```python
from build123d import *

# Parameters (mm, degrees)
SKETCH1_R                = 1.5
SKETCH1_R_2              = 2.5
BOSS_EXTRUDE1_DEPTH      = 20
SKETCH2_W                = 8.1
SKETCH2_H                = 20
SKETCH2_W_2              = 5.2
SKETCH2_W_3              = 5.1
CUT_EXTRUDE1_DEPTH       = 20
CUT_EXTRUDE1_DEPTH_BACK  = 20
CUT_EXTRUDE2_DEPTH       = 9
BOSS_EXTRUDE2_DEPTH      = 11.9
SKETCH5_R                = 3
BOSS_EXTRUDE3_DEPTH      = 5
CUT_EXTRUDE6_DEPTH       = 1
SKETCH13_R               = 2.5
CUT_EXTRUDE7_DEPTH       = 4
BOSS_EXTRUDE4_DEPTH      = 3
CUT_EXTRUDE9_DEPTH       = 3
SKETCH17_W               = 9
SKETCH17_H               = 3.569322199
CUT_EXTRUDE11_DEPTH      = 3
SKETCH18_W               = 5.770974844
SKETCH18_H               = 0.772936936
BOSS_EXTRUDE5_DEPTH      = 6.9
BOSS_EXTRUDE5_DEPTH_BACK = 1
SKETCH19_W               = 5.1
SKETCH19_H               = 16.397725614
CUT_EXTRUDE12_DEPTH      = 0.301495
SKETCH20_W               = 5
SKETCH20_H               = 12.419235667
CUT_EXTRUDE13_DEPTH      = 10
BOSS_EXTRUDE6_DEPTH      = 2
SKETCH23_W               = 4.9
SKETCH23_H               = 6
BOSS_EXTRUDE7_DEPTH      = 4
SKETCH22_R               = 1
CUT_EXTRUDE15_DEPTH      = 8
BOSS_EXTRUDE8_DEPTH      = 2
SKETCH14_R               = 1.5
CUT_EXTRUDE8_DEPTH       = 10.1
CUT_EXTRUDE17_DEPTH      = 8.1
CUT_EXTRUDE17_DEPTH_BACK = 2
CUT_EXTRUDE18_DEPTH      = 2
CUT_EXTRUDE20_DEPTH      = 5.2
SKETCH30_W               = 6.9
SKETCH30_H               = 20
CUT_EXTRUDE21_DEPTH      = 0.283797
CUT_EXTRUDE22_REACH      = 91.699
SKETCH31_W               = 2
SKETCH31_H               = 11.022421386
CUT_EXTRUDE23_DEPTH      = 7
CUT_EXTRUDE24_DEPTH      = 21
SKETCH34_W               = 60.526432738
SKETCH34_H               = 58.455185991
CUT_EXTRUDE25_DEPTH      = 21


with BuildPart() as part:
    # Sketch1 → Boss-Extrude1 (new body)
    with BuildSketch(Plane(origin=(0, 0, 0), x_dir=(0, 0, -1), z_dir=(1, 0, 0))):
        with BuildLine():
            ThreePointArc((9.765353557, 20.116545894), (0, 32.270117322), (-9.765353557, 20.116545894))
            ThreePointArc((-9.765353557, 20.116545894), (-5.132645827, -18.047253777), (-7.88740095, -56.392382678))
            ThreePointArc((-7.88740095, -56.392382678), (0, -65.729882678), (7.88740095, -56.392382678))
            ThreePointArc((7.88740095, -56.392382678), (5.132645827, -18.047253777), (9.765353557, 20.116545894))
        make_face()
        with Locations((0, 22.270117322)):
            Circle(SKETCH1_R, mode=Mode.SUBTRACT)
        with Locations((0, -57.729882678)):
            Circle(SKETCH1_R_2, mode=Mode.SUBTRACT)
    extrude(amount=BOSS_EXTRUDE1_DEPTH)

    # Sketch2 → Cut-Extrude1 (cut, two sides)
    with BuildSketch(Plane.XY) as cut_extrude1_sk:
        with Locations((4.05, -55.729882678)):
            Rectangle(SKETCH2_W, SKETCH2_H)
        with Locations((17.4, -55.729882678)):
            Rectangle(SKETCH2_W_2, SKETCH2_H)
        with Locations((5.55, 22.270117322)):
            Rectangle(SKETCH2_W_3, SKETCH2_H)
    extrude(amount=CUT_EXTRUDE1_DEPTH, mode=Mode.SUBTRACT)
    extrude(cut_extrude1_sk.sketch, amount=-CUT_EXTRUDE1_DEPTH_BACK, mode=Mode.SUBTRACT)

    # Sketch3 → Cut-Extrude2 (cut)
    with BuildSketch(Plane.ZY.offset(-8.1)):
        with BuildLine():
            Line((8.5, 22.270117322), (8.5, 40.909533312))
            Line((8.5, 40.909533312), (-17.52872033, 40.909533312))
            Line((-17.52872033, 40.909533312), (-17.52872033, 13.770117322))
            Line((-17.52872033, 13.770117322), (0, 13.770117322))
            ThreePointArc((0, 13.770117322), (6.01040764, 16.259709682), (8.5, 22.270117322))
        make_face()
    extrude(amount=-CUT_EXTRUDE2_DEPTH, mode=Mode.SUBTRACT)

    # Sketch4 → Boss-Extrude2 (add, through all)
    with BuildSketch(Plane.ZY.offset(-8.1)):
        Polygon((8.5, 27.537944199), (8.283796844, 12.741558936), (10.283796844, 12.741558936), (10.283796844, 27.537944199), align=None)
    extrude(amount=-BOSS_EXTRUDE2_DEPTH)

    # Sketch5 → Boss-Extrude3 (add)
    with BuildSketch(Plane.ZY.offset(-8.1)):
        with BuildLine():
            Line((8.145156861, 11.968622), (8.447845456, 23.968622))
            Line((8.447845456, 23.968622), (9.854698466, 23.968622))
            Line((9.854698466, 23.968622), (15.022421386, 23.968622))
            ThreePointArc((15.022421386, 23.968622), (21.022421386, 17.968622), (15.022421386, 11.968622))
            Line((15.022421386, 11.968622), (8.145156861, 11.968622))
        make_face()
        with Locations((15.022421386, 17.968622)):
            Circle(SKETCH5_R, mode=Mode.SUBTRACT)
    extrude(amount=-BOSS_EXTRUDE3_DEPTH)

    # Sketch12 → Cut-Extrude6 (cut)
    with BuildSketch(Plane(origin=(13.1, 0, 0), x_dir=(0, 0, -1), z_dir=(1, 0, 0))):
        Polygon((-13.902900694, 14.968622), (-13.902900694, 12.968622), (-15.902900694, 12.968622), (-15.902900694, 14.968622), (-15.902900694, 15.294296094), (-13.902900694, 15.294296094), align=None)
    extrude(amount=-CUT_EXTRUDE6_DEPTH, mode=Mode.SUBTRACT)

    # Sketch13 → Cut-Extrude7 (cut)
    with BuildSketch(Plane.ZY.offset(-17.1)):
        with Locations((0, 22.270117322)):
            Circle(SKETCH13_R)
    extrude(amount=-CUT_EXTRUDE7_DEPTH, mode=Mode.SUBTRACT)

    # Sketch15 → Boss-Extrude4 (add)
    with BuildSketch(Plane.ZY):
        Polygon((10, 22.270117322), (10, 11.968622), (8.145156861, 11.968622), (7.595672539, 11.968622), align=None)
    extrude(amount=-BOSS_EXTRUDE4_DEPTH)

    # Sketch16 → Cut-Extrude9 (cut)
    with BuildSketch(Plane(origin=(20, 0, 0), x_dir=(0, 0, -1), z_dir=(1, 0, 0))):
        with BuildLine():
            Line((-10.283796844, 23.968622), (-9.854698466, 23.968622))
            ThreePointArc((-9.854698466, 23.968622), (-9.349264901, 25.818531871), (-8.5, 27.537944199))
            Line((-8.5, 27.537944199), (-10.283796844, 27.537944199))
            Line((-10.283796844, 27.537944199), (-10.283796844, 23.968622))
        make_face()
    extrude(amount=-CUT_EXTRUDE9_DEPTH, mode=Mode.SUBTRACT)

    # Sketch17 → Cut-Extrude11 (cut)
    with BuildSketch(Plane.XY.offset(10.283796844)):
        with Locations((12.6, 25.7532831)):
            Rectangle(SKETCH17_W, SKETCH17_H)
    extrude(amount=-CUT_EXTRUDE11_DEPTH, mode=Mode.SUBTRACT)

    # Sketch18 → Boss-Extrude5 (add, two sides)
    with BuildSketch(Plane(origin=(13.1, 0, 0), x_dir=(0, 0, -1), z_dir=(1, 0, 0))) as boss_extrude5_sk:
        with Locations((-7.398309422, 12.355090468)):
            Rectangle(SKETCH18_W, SKETCH18_H)
    extrude(amount=BOSS_EXTRUDE5_DEPTH)
    extrude(boss_extrude5_sk.sketch, amount=-BOSS_EXTRUDE5_DEPTH_BACK)

    # Sketch19 → Cut-Extrude12 (cut)
    with BuildSketch(Plane(origin=(0, 12.270117322, 0), x_dir=(1, 0, 0), z_dir=(0, 1, 0))):
        with Locations((5.55, 0)):
            Rectangle(SKETCH19_W, SKETCH19_H)
    extrude(amount=-CUT_EXTRUDE12_DEPTH, mode=Mode.SUBTRACT)

    # Sketch20 → Cut-Extrude13 (cut)
    with BuildSketch(Plane.ZY.offset(-17.1)):
        with Locations((0, 28.479735156)):
            Rectangle(SKETCH20_W, SKETCH20_H)
    extrude(amount=-CUT_EXTRUDE13_DEPTH, mode=Mode.SUBTRACT)

    # Sketch21 → Boss-Extrude6 (add)
    with BuildSketch(Plane.ZY.offset(-17.1)):
        with BuildLine():
            Line((-8.473151119, 13.770117322), (0.278481736, 12.273995678))
            ThreePointArc((0.278481736, 12.273995678), (9.936881703, 21.148341047), (2.5, 31.952575688))
            Line((2.5, 31.952575688), (2.5, 22.270117322))
            ThreePointArc((2.5, 22.270117322), (0, 19.770117322), (-2.5, 22.270117322))
            Line((-2.5, 22.270117322), (-2.5, 31.952575688))
            ThreePointArc((-2.5, 31.952575688), (-8.522477621, 27.501501002), (-9.765353557, 20.116545894))
            ThreePointArc((-9.765353557, 20.116545894), (-9.093560923, 16.948562662), (-8.473151119, 13.770117322))
        make_face()
    extrude(amount=BOSS_EXTRUDE6_DEPTH)

    # Sketch23 → Boss-Extrude7 (add)
    with BuildSketch(Plane.XY.offset(10.283796844)):
        with Locations((17.55, 26.968622)):
            Rectangle(SKETCH23_W, SKETCH23_H)
    extrude(amount=-BOSS_EXTRUDE7_DEPTH)

    # Sketch22 → Cut-Extrude15 (cut)
    with BuildSketch(Plane.XY.offset(10.283796844)):
        with Locations((17.55, 26.870117322)):
            Circle(SKETCH22_R)
    extrude(amount=-CUT_EXTRUDE15_DEPTH, mode=Mode.SUBTRACT)

    # Sketch24 → Boss-Extrude8 (add)
    with BuildSketch(Plane.ZY.offset(-8.1)):
        with BuildLine():
            Line((5.147845456, 19.737443909), (5.147845456, 15.506265819))
            Line((5.147845456, 15.506265819), (8.447845456, 15.506265819))
            Line((8.447845456, 15.506265819), (8.447845456, 23.968622))
            add(Edge.make_bspline(
                [(8.447845456, 23.968622), (5.147845456, 23.968622), (5.147845456, 19.737443909)],
                knots=[3.141592654, 3.141592654, 3.141592654, 4.71238898, 4.71238898, 4.71238898], degree=2, weights=[1, 0.707106781, 1]))
        make_face()
    extrude(amount=-BOSS_EXTRUDE8_DEPTH)

    # Sketch14 → Cut-Extrude8 (cut)
    with BuildSketch(Plane.ZY):
        with Locations((7.532575614, 18.331804915)):
            Circle(SKETCH14_R)
    extrude(amount=-CUT_EXTRUDE8_DEPTH, mode=Mode.SUBTRACT)

    # Sketch25 → Cut-Extrude17 (cut, two sides)
    with BuildSketch(Plane.ZY.offset(-8.1)) as cut_extrude17_sk:
        with BuildLine():
            Line((12, -45.729882678), (8.346153846, -36.960651908))
            ThreePointArc((8.346153846, -36.960651908), (6.973852263, -42.37911752), (2.5, -45.729882678))
            Line((2.5, -45.729882678), (2.5, -53.227383372))
            ThreePointArc((2.5, -53.227383372), (0, -62.879882678), (-2.5, -53.227383372))
            Line((-2.5, -53.227383372), (-2.5, -45.729882678))
            ThreePointArc((-2.5, -45.729882678), (-6.973852263, -42.37911752), (-8.346153846, -36.960651908))
            Line((-8.346153846, -36.960651908), (-12, -45.729882678))
            Line((-12, -45.729882678), (-12, -57.729882678))
            ThreePointArc((-12, -57.729882678), (0, -69.729882678), (12, -57.729882678))
            Line((12, -57.729882678), (12, -45.729882678))
        make_face()
    extrude(amount=CUT_EXTRUDE17_DEPTH, mode=Mode.SUBTRACT)
    extrude(cut_extrude17_sk.sketch, amount=-CUT_EXTRUDE17_DEPTH_BACK, mode=Mode.SUBTRACT)

    # Sketch26 → Cut-Extrude18 (cut)
    with BuildSketch(Plane(origin=(20, 0, 0), x_dir=(0, 0, -1), z_dir=(1, 0, 0))):
        with BuildLine():
            Line((-7.209968303, 15.085404497), (-10.283796844, 15.085404497))
            Line((-10.283796844, 15.085404497), (-10.283796844, 17.085404497))
            Line((-10.283796844, 17.085404497), (-7.209968303, 17.085404497))
            ThreePointArc((-7.209968303, 17.085404497), (-4.010444351, 15.949526558), (-2.243391617, 13.050441039))
            ThreePointArc((-2.243391617, 13.050441039), (0.649659998, -12.257973546), (0.397031114, -37.729953741))
            Line((0.397031114, -37.729953741), (-1.608183929, -37.729953741))
            ThreePointArc((-1.608183929, -37.729953741), (-1.343036313, -12.450773719), (-4.206611504, 12.667092093))
            ThreePointArc((-4.206611504, 12.667092093), (-5.281990934, 14.405678614), (-7.209968303, 15.085404497))
        make_face()
    extrude(amount=-CUT_EXTRUDE18_DEPTH, mode=Mode.SUBTRACT)

    # Sketch29 → Cut-Extrude20 (cut)
    with BuildSketch(Plane(origin=(20, 0, 0), x_dir=(0, 0, -1), z_dir=(1, 0, 0))):
        with BuildLine():
            Line((8, -37.729882678), (8.140336581, -37.729882678))
            Line((8.140336581, -37.729882678), (8.140336581, -45.937498976))
            Line((8.140336581, -45.937498976), (-15.754893946, -45.937498976))
            Line((-15.754893946, -45.937498976), (-15.754893946, -37.729882678))
            Line((-15.754893946, -37.729882678), (-8, -37.729882678))
            ThreePointArc((-8, -37.729882678), (0, -45.729882678), (8, -37.729882678))
        make_face()
    extrude(amount=-CUT_EXTRUDE20_DEPTH, mode=Mode.SUBTRACT)

    # Sketch30 → Cut-Extrude21 (cut)
    with BuildSketch(Plane.XY.offset(10.283796844)):
        with Locations((16.55, 21.968622)):
            Rectangle(SKETCH30_W, SKETCH30_H)
    extrude(amount=-CUT_EXTRUDE21_DEPTH, mode=Mode.SUBTRACT)

    # Sketch31 → Cut-Extrude22 (cut, up to next)
    with BuildSketch(Plane(origin=(0, 23.968622, 0), x_dir=(1, 0, 0), z_dir=(0, 1, 0)), mode=Mode.PRIVATE) as cut_extrude22_sk1:
        with Locations((9.1, -15.511210693)):
            Rectangle(SKETCH31_W, SKETCH31_H)
    cut_extrude22_tool1 = extrude(cut_extrude22_sk1.sketch, amount=-CUT_EXTRUDE22_REACH, mode=Mode.PRIVATE) & part.part
    add(cut_extrude22_tool1.solids().sort_by_distance((9.1, 23.968622, 15.511211))[0], mode=Mode.SUBTRACT)

    # Sketch32 → Cut-Extrude23 (cut)
    with BuildSketch(Plane.ZY.offset(-8.1)):
        Polygon((-8.473151119, 13.770117322), (-8.473151119, 5.401068454), (5.147845456, 15.506265819), align=None)
    extrude(amount=-CUT_EXTRUDE23_DEPTH, mode=Mode.SUBTRACT)

    # Sketch33 → Cut-Extrude24 (cut, through all)
    with BuildSketch(Plane(origin=(20, 0, 0), x_dir=(0, 0, -1), z_dir=(1, 0, 0))):
        Polygon((-9.30475326, -22.954882678), (-9.30475326, -27.954882678), (8.892389241, -27.954882678), (8.892389241, -22.954882678), (8.892389241, -17.954882678), (-9.30475326, -17.954882678), align=None)
    extrude(amount=-CUT_EXTRUDE24_DEPTH, mode=Mode.SUBTRACT)

    # Sketch34 → Cut-Extrude25 (cut, through all)
    with BuildSketch(Plane(origin=(20, 0, 0), x_dir=(0, 0, -1), z_dir=(1, 0, 0))):
        with Locations((-5.515206789, -53.322694673)):
            Rectangle(SKETCH34_W, SKETCH34_H)
    extrude(amount=-CUT_EXTRUDE25_DEPTH, mode=Mode.SUBTRACT)


solid = part.part
```
Verification items for the finished model (mm, model axes). A direction names the side the tool comes from. Round coordinates to 2 decimals unless told otherwise and drop trailing zeros. Order: outer loops, then holes, each group sorted by start corner. A loop starts at its lowest first (then second) coordinate and runs counter-clockwise, first axis right, second up.
1) Draft check along X on faces 5 (the flat face through (3, 20, 0)), 6 (the flat face through (0, 8, 0)), 7 (the flat face through (1, 11.969, 9)). Enter one of: +X half, -X half, draft (parallel to the pull), parting line (faces both ways), or undercut.
Geometry says:
face 5: undercut
face 6: -X half
face 7: draft
2) Material ranges on line 1 (Y direction, x = 0.8, z = 0); line 2 (X direction, y = 20, z = 4); line 3 (Y direction, x = 8, z = 1.5), recorded low to high.
Geometry says:
line 1: y = -17.95 to 20.77, 23.77 to 32.27
line 2: x = 0 to 3, 15.1 to 20
line 3: y = -17.95 to 11.97
3) Tool access check on faces 1 (the flat face through (13.1, 21, 17)), 2 (the flat face through (12, 23.969, 11)), 3 (the flat face through (18, 28, 2.5)), 4 (the flat face through (10.1, 18, 8)). Record the directions out of +Z, -Z, +X, -X, +Y, -Y that give a thin tool (end or side, any length) a straight path to the whole face; none if there is none.
Geometry says:
face 1: +Z, +X, +Y, -Y
face 2: +Z, -Z, +Y
face 3: +X, +Y
face 4: -X
4) Cross-section at A-A, the plane y = -0.5. Record the cut outline in (x, z).
Geometry says:
outline: (0, -6.34) - (20, -6.34) - (20, 0.3) - (18, 0.3) - (18, 2.31) - (20, 2.31) - (20, 6.34) - (0, 6.34) - close
5) Cross-section at D-D, the plane y = -7.5. Record the cut outline in (x, z).
Geometry says:
outline: (0, -5.67) - (20, -5.67) - (20, -0.35) - (18, -0.35) - (18, 1.66) - (20, 1.66) - (20, 5.67) - (0, 5.67) - close
6) Depth check by flat-ended pin: pin 1 (1 mm diameter, centred on x = 18, y = 7, fed in from +Z); pin 2 (2 mm diameter, centred on x = 1, z = 9.5, fed in from -Y); pin 3 (5.5 mm diameter, centred on y = 17.97, z = 15.02, fed in from +X); pin 4 (1.5 mm diameter, centred on x = 17, y = 28, fed in from +Z). Enter the tip coordinate at first touch or a pass-through.
Geometry says:
pin 1: stops at z = 7.4
pin 2: stops at y = 11.97
pin 3: passes through
pin 4: stops at z = 10
7) Cross-section at C-C, the plane y = 9.5. Record the cut outline in (x, z).
Geometry says:
outline: (0, -7.72) - (8.1, -7.72) - (8.1, -2.95) - (15.1, -2.95) - (15.1, -7.72) - (20, -7.72) - (20, 1.65) - (18, 1.65) - (18, 3.67) - (20, 3.67) - (20, 7.72) - (0, 7.72) - close
8) Cross-section at B-B, the plane z = 11. Record the cut outline in (x, y).
Geometry says:
outline: (10.1, 11.97) - (13.1, 11.97) - (13.1, 23.97) - (10.1, 23.97) - close
